from build123d import *


with BuildPart() as part:
    # Sketch1 → Revolve3 (revolve)
    with BuildSketch(Plane.XY, mode=Mode.PRIVATE) as revolve3_sk:
        with BuildLine():
            Line((-17.399, 0), (-17.399, -40.64))
            Line((-17.399, -40.64), (-19.269565144, -40.64))
            Line((-19.269565144, -40.64), (-19.269565144, 0))
            Line((-19.269565144, 0), (-20.32, 0))
            ThreePointArc((-20.32, 0), (-16.432425265, 89.23807563), (-4.799156969, 177.8))
            Line((-4.799156969, 177.8), (-1.833166816, 177.8))
            ThreePointArc((-1.833166816, 177.8), (-13.500113667, 89.240034686), (-17.399, 0))
        make_face()
    revolve(revolve3_sk.sketch.rotate(Axis((0, 203.2, 0), (0, -1, 0)), 270), axis=Axis((0, 203.2, 0), (0, -1, 0)))


solid = part.part
Verification items for the finished model (mm, model axes). A direction names the side the tool comes from. Coordinates: 2 decimals unless noted, no trailing zeros. Order: outer loops, then holes, each group sorted by start corner. A loop starts at its lowest first (then second) coordinate and runs counter-clockwise, first axis right, second up.
Item 1: Material ranges on L1, parallel to X at y = -15, z = 0; L2, parallel to Z at x = -14, y = 44.5; L3, parallel to X at y = 31.5, z = 14.5, recorded low to high.
Filled in:
L1: x = -19.27 to -17.4, 17.4 to 19.27
L2: z = -13.36 to -8.6, 8.6 to 13.36
L3: x = -13.54 to -8.71, 8.71 to 13.54
Item 2: Section check A-A, the plane y = -24. Enter the section's corners in (x, z).
Filled in:
outline: circle Ø38.54 at (0, 0); hole circle Ø34.8 at (0, 0)
Item 3: Depth check by flat-ended pin: pin 1 (3 mm diameter, centred on y = 64.5, z = -2, fed in from +X); pin 2 (3 mm diameter, centred on y = 93, z = 16, fed in from +X); pin 3 (10 mm diameter, centred on y = 65, z = -8, fed in from +X). Enter the tip coordinate at first touch or a pass-through.
Filled in:
pin 1: stops at x = 18.33
pin 2: stops at x = 7.01
pin 3: stops at x = 18.07
Item 4: Release check for a two-part mould opening along X. For faces 1 (the face through (-14.4, -40.64, 10.1)), 2 (the face through (10.587, -20.604, -13.807)), 3 (the face through (-5.79, -20.04, 18.38)) record: +X half, -X half, draft (parallel to the pull), parting line (faces both ways), or undercut.
Filled in:
face 1: draft
face 2: undercut
face 3: parting line
Item 5: Access from +Z, -Z, +X, -X, +Y, -Y to the whole of each face (thin tool, end or side, straight path). Record for faces 4 (the face through (2, 177.8, 0)), 5 (the face through (7.4, 0, -18)).
Filled in:
face 4: +Z, -Z, +X, -X, +Y
face 5: -Y
